Source: CAD feature listing. Evaluate the final solid. Frame: model axes, mm. Face numbers are marked on the shaded views. A direction names the side the tool comes from. Coordinates: 2 decimals unless noted, no trailing zeros. Write each loop counter-clockwise with the first axis right and the second up, starting at its lowest first coordinate (ties: lowest second). Pieces come first, ordered by that corner, then holes. Notation, with made-up numbers: (-36, 11) - (-26, 11) arc R18 cw to (-26, 22) - close; hole circle Ø7 at (-2.5, -30.5). An arc over 180 degrees is marked (long way). One line per question, with ' | ' between items.
from build123d import *

# Parameters (mm, degrees)
SKETCH1_R               = 50
SKETCH1_R_2             = 20
BOSS_EXTRUDE1_DEPTH     = 15
SKETCH1_3_R             = 20
SKETCH1_3_R_2           = 15
BOSS_EXTRUDE2_DEPTH     = 40
SKETCH2_W               = 6
SKETCH2_H               = 4
CUT_EXTRUDE1_DEPTH      = 80
CUT_EXTRUDE2_DEPTH      = 80
CUT_EXTRUDE2_DEPTH_BACK = 80
SKETCH3_W               = 10
SKETCH3_H               = 10


with BuildPart() as part:
    # Sketch1 → Boss-Extrude1 (new body)
    with BuildSketch(Plane.XY):
        Circle(SKETCH1_R)
        Circle(SKETCH1_R_2, mode=Mode.SUBTRACT)
    extrude(amount=BOSS_EXTRUDE1_DEPTH)

    # Sketch1<3> → Boss-Extrude2 (add)
    with BuildSketch(Plane.XY):
        Circle(SKETCH1_3_R)
        Circle(SKETCH1_3_R_2, mode=Mode.SUBTRACT)
    extrude(amount=BOSS_EXTRUDE2_DEPTH)

    # Sketch2 → Cut-Extrude1 (cut)
    with BuildSketch(Plane.XY):
        with Locations((0, 16.5)):
            Rectangle(SKETCH2_W, SKETCH2_H)
    extrude(amount=CUT_EXTRUDE1_DEPTH, mode=Mode.SUBTRACT)

    # Sketch3 → Cut-Extrude2 (cut, two sides: drawn at the far end of the back side and taken through both)
    with BuildSketch(Plane(origin=(0, 0, 0), x_dir=(1, 0, 0), z_dir=(0, 1, 0)).offset(-CUT_EXTRUDE2_DEPTH_BACK)):
        with Locations((0, -5)):
            Rectangle(SKETCH3_W, SKETCH3_H)
    extrude(amount=CUT_EXTRUDE2_DEPTH + CUT_EXTRUDE2_DEPTH_BACK, mode=Mode.SUBTRACT)


solid = part.part
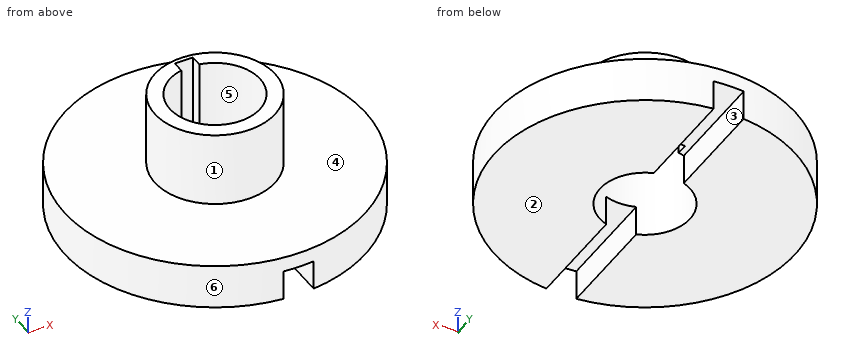
Item 1: Mould query, pull axis X, two halves, no side actions, for the marked faces 4, 5 and 6. Classes: pulls with the +X half, pulls with the -X half, needs draft (parallel to the pull), parting line crosses it, or undercut.
Check sheet entries:
face 4: needs draft | face 5: undercut | face 6: parting line crosses it
Item 2: Cut plane B-B on y = 0. Return loops of the section in (x, z), and give its area (3 significant figures).
Check sheet entries:
outline: (-50, 0) - (-15, 0) - (-15, 40) - (-20, 40) - (-20, 15) - (-50, 15) - close; (15, 0) - (50, 0) - (50, 15) - (20, 15) - (20, 40) - (15, 40) - close | area: 1,300 mm²
Item 3: Access query for the marked faces 1, 2 and 3. Directions: +Z, -Z, +X, -X, +Y, -Y. A direction counts if a zero-diameter tool reaches every point of the face in a straight line with its end or side. Return the directions, or none.
Check sheet entries:
face 1: +Z | face 2: -Z, +X, -X, +Y, -Y | face 3: -Z, +Y, -Y
Item 4: Cut plane C-C on z = 5. Return loops of the section in (x, y), and give its area (3 significant figures).
Check sheet entries:
outline: (-5, -49.75) - (-5, -14.14) arc R15 cw to (-5, 14.14) - (-5, 49.75) arc R50 ccw to start; (5, -49.75) arc R50 ccw to (5, 49.75) - (5, 14.14) arc R15 cw to (5, -14.14) - close | area: 6,440 mm²
Item 5: Pin query (flat end, axial travel): pin 1 Ø5 at (x, y) = (-0.5, 28) entering from -Z; pin 2 Ø1.9 at (y, z) = (16, 20.5) entering from -X; pin 3 Ø4 at (y, z) = (16, 28) entering from +X. Return the tip coordinate at first contact, or that it passes through.
Check sheet entries:
pin 1: z = 10 | pin 2: x = -13.17 | pin 3: x = 14.28
Item 6: Cut plane A-A on x = 0. Return loops of the section in (y, z).
Check sheet entries:
outline: (-50, 10) - (-15, 10) - (-15, 40) - (-20, 40) - (-20, 15) - (-50, 15) - close; (18.5, 10) - (50, 10) - (50, 15) - (20, 15) - (20, 40) - (18.5, 40) - close
Item 7: Ray query, line 1 along Y through (x, z) = (0, 29.5); line 2 along Z through (x, y) = (42, -19.5); line 3 along Y through (x, z) = (-12, 34). Return the intervals inside material, ascending. Write a range as [from, to].
Check sheet entries:
line 1: [-20, -15], [18.5, 20] | line 2: [0, 15] | line 3: [-16, -9], [9, 16]
Item 8: Cut plane D-D on z = 11.5. Return loops of the section in (x, y).
Check sheet entries:
outline: circle Ø100 at (0, 0); hole (-3, 14.7) arc R15 ccw (long way) to (3, 14.7) - (3, 18.5) - (-3, 18.5) - close
